Work out the finished part from the listing and answer in its coordinate system (mm). Face numbers are marked on the shaded views. A direction names the side the tool comes from. Round coordinates to 2 decimals unless told otherwise and drop trailing zeros. Order: outer loops, then holes, each group sorted by start corner. A loop starts at its lowest first (then second) coordinate and runs counter-clockwise, first axis right, second up. Notation, with made-up numbers: M 21.25,-33.5 L 47.25,-33.5 A19 ccw 47.25,-13.5 Z; hole C 12,-13 d9. An arc over 180 degrees is marked long. Return JSON: item names as keys, results as strings.
from build123d import *

# Parameters (mm, degrees)
SKETCH1_R      = 4.0005
SKETCH1_R_2    = 0.79375
EXTRUDE1_DEPTH = 7.4422
SKETCH4_W      = 3.556
SKETCH4_H      = 6.4516
EXTRUDE2_DEPTH = 9.525


with BuildPart() as part:
    # Sketch1 → Extrude1 (new body)
    with BuildSketch(Plane(origin=(0, 0, 0), x_dir=(0, 0, -1), z_dir=(1, 0, 0))):
        Circle(SKETCH1_R)
        Circle(SKETCH1_R_2, mode=Mode.SUBTRACT)
    extrude(amount=-EXTRUDE1_DEPTH)

    # Sketch4 → Extrude2 (add)
    with BuildSketch(Plane.ZY.offset(7.4422)):
        Rectangle(SKETCH4_W, SKETCH4_H)
    extrude(amount=EXTRUDE2_DEPTH)


solid = part.part
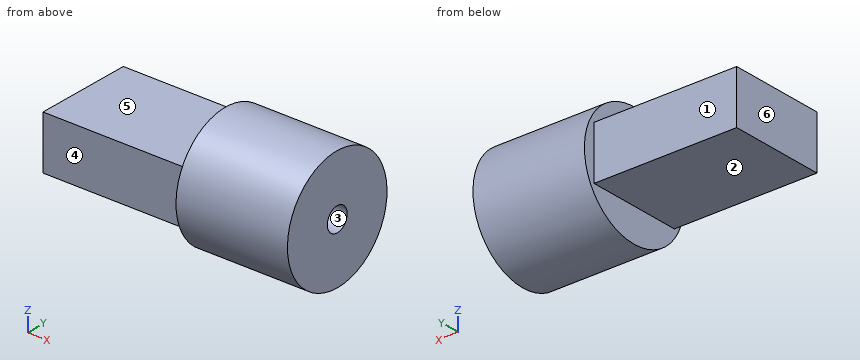
Item 1: Find section A-A (z = 0). Determine the outline of the cut face in (x, y).
Output:
{"outline": "M -16.97,-3.23 L -7.44,-3.23 L -7.44,-4 L 0,-4 L 0,-0.79 L -7.44,-0.79 L -7.44,0.79 L 0,0.79 L 0,4 L -7.44,4 L -7.44,3.23 L -16.97,3.23 Z"}
Item 2: Each of these flat-tipped pins is pushed along its axis until it touches: pin 1 (1 mm diameter, centred on y = 0, z = 0, fed in from +X); pin 2 (3 mm diameter, centred on x = -12.5, z = 0.5, fed in from +Y); pin 3 (1.8 mm diameter, centred on x = -10.5, z = -1, fed in from -Y). Where does it stop, or does it pass through?
Output:
{"pin 1": "stops at x = -7.44", "pin 2": "stops at y = 3.23", "pin 3": "stops at y = -3.23"}
Item 3: Which of the six approach directions +Z, -Z, +X, -X, +Y, -Y give full straight-line access (tool end or side, diameter ignored) to the marked faces 4, 5 and 6?
Output:
{"face 4": "+Z, -Z, -X, -Y", "face 5": "+Z, -X, +Y, -Y", "face 6": "+Z, -Z, -X, +Y, -Y"}
Item 4: Consider line 1 along Y through (x, z) = (-2.25, 0); line 2 along X through (y, z) = (2, -2.25); line 3 along Z through (x, y) = (-1, 0.25). Determine where each line is inside the solid, lowest interval first. Write a range as [from, to].
Output:
{"line 1": "y = [-4, -0.79], [0.79, 4]", "line 2": "x = [-7.44, 0]", "line 3": "z = [-3.99, -0.75], [0.75, 3.99]"}
Item 5: The mould has two halves that part along Z. Classify the marked faces 1, 2 and 3: pulls with the +Z half, pulls with the -Z half, needs draft (parallel to the pull), parting line crosses it, or undercut.
Output:
{"face 1": "needs draft", "face 2": "pulls with the -Z half", "face 3": "undercut"}
Item 6: Find section C-C (x = -14.75). Determine the outline of the cut face in (y, z).
Output:
{"outline": "M -3.23,-1.78 L 3.23,-1.78 L 3.23,1.78 L -3.23,1.78 Z"}
Item 7: Find section D-D (x = -2.25). Determine the outline of the cut face in (y, z).
Output:
{"outline": "C 0,0 d8; hole C 0,0 d1.59"}
Item 8: Find section B-B (y = 0). Determine the outline of the cut face in (x, z), plus the area to 3 significant figures.
Output:
{"outline": "M -16.97,-1.78 L -7.44,-1.78 L -7.44,-4 L 0,-4 L 0,-0.79 L -7.44,-0.79 L -7.44,0.79 L 0,0.79 L 0,4 L -7.44,4 L -7.44,1.78 L -16.97,1.78 Z", "area": "81.6 mm^2"}
